Job drawing, mm, ordinate dimensions from the low corner. One solid piece. Give positions to 0.01 mm unless a question says otherwise; leave off trailing zeros. Order: outer loops, then holes, each group sorted by start corner. A loop starts at its lowest first (then second) coordinate and runs counter-clockwise, first axis right, second up.
1. Probe line 1 (Z direction, x = 31, y = 2.4); line 2 (X direction, y = 0.35, z = 20.5); line 3 (X direction, y = 1.85, z = 13) (3 decimals). List the from-to ranges inside material, lowest first.
2. Slice it at D-D on x = 9. List the corners of the cut face in (y, z).
3. Drop flat-ended pins along their axis: pin 1 Ø0.9 at (y, z) = (1, 14) entering from +X; pin 2 Ø1.5 at (x, y) = (25.5, 2.5) entering from -Z; pin 3 Ø1.5 at (y, z) = (1.5, 30) entering from +X. Give the stop position or say it passes through.
4. Slice it at C-C on y = 0.85. List the corners of the cut face in (x, z).
5. Slice it at B-B on z = 11. List the corners of the cut face in (x, y).
6. Slice it at A-A on x = 20. List the corners of the cut face in (y, z).
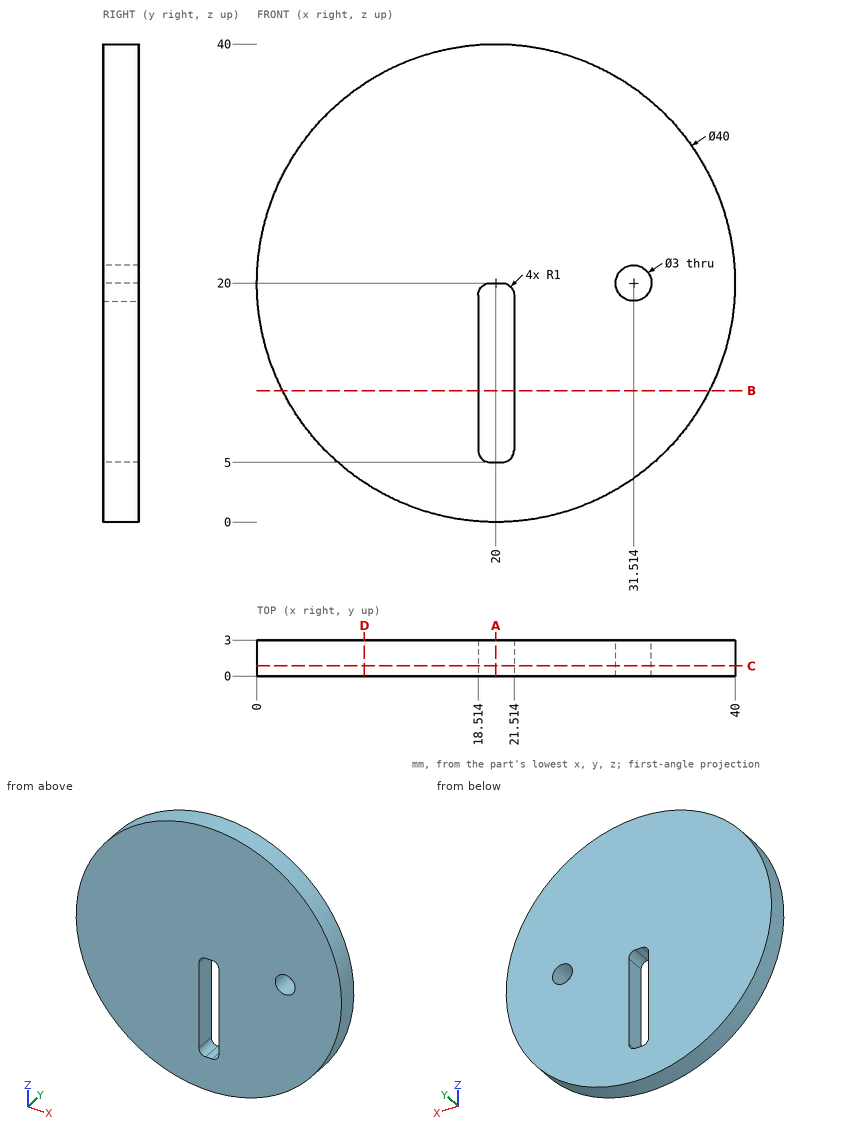
Data:
1. line 1: z = 3.3 to 18.59, 21.41 to 36.7
1. line 2: x = 0.01 to 30.1, 32.93 to 39.99
1. line 3: x = 1.265 to 18.514, 21.514 to 38.735
2. outline: (0, 3.3) - (3, 3.3) - (3, 36.7) - (0, 36.7) - close
3. pin 1: stops at x = 39.21
3. pin 2: stops at z = 0.57
3. pin 3: stops at x = 37.73
4. outline: circle Ø40 at (20, 20); hole (18.51, 6) arc R1 ccw to (19.51, 5) - (20.51, 5) arc R1 ccw to (21.51, 6) - (21.51, 19) arc R1 ccw to (20.51, 20) - (19.51, 20) arc R1 ccw to (18.51, 19) - close; hole circle Ø3 at (31.51, 20)
5. outline: (2.14, 0) - (18.51, 0) - (18.51, 3) - (2.14, 3) - close; (21.51, 0) - (37.86, 0) - (37.86, 3) - (21.51, 3) - close
6. outline: (0, 0) - (3, 0) - (3, 5) - (0, 5) - close; (0, 20) - (3, 20) - (3, 40) - (0, 40) - close
